```python
from build123d import *

# Parameters (mm, degrees)
ESBO_O1_R                = 18
RESSALTO_EXTRUS_O1_DEPTH = 3
RESSALTO_EXTRUS_O2_START = 5
RESSALTO_EXTRUS_O2_DEPTH = 5
RESSALTO_EXTRUS_O3_START = 2
RESSALTO_EXTRUS_O3_DEPTH = 2


with BuildPart() as part:
    # Esbo_o1 → Ressalto-extrus_o1 (new body)
    with BuildSketch(Plane.XY):
        with BuildLine():
            ThreePointArc((18, 0), (0, -18), (-18, 0))
            Line((-18, 0), (-18, 10.816653826))
            ThreePointArc((-18, 10.816653826), (-5.61248608, -20.236106345), (21, 0))
            ThreePointArc((21, 0), (20.236106345, 5.61248608), (18, 10.816653826))
            Line((18, 10.816653826), (18, 0))
        make_face()
        with BuildLine():
            Line((-18, 10.816653826), (-18, 0))
            ThreePointArc((-18, 0), (0, 18), (18, 0))
            Line((18, 0), (18, 10.816653826))
            ThreePointArc((18, 10.816653826), (0, 21), (-18, 10.816653826))
        make_face()
        Circle(ESBO_O1_R)
    extrude(amount=-RESSALTO_EXTRUS_O1_DEPTH)

    # Esbo_o1_3 → Ressalto-extrus_o2 (add)
    with BuildSketch(Plane.XY.offset(RESSALTO_EXTRUS_O2_START)):
        with BuildLine():
            ThreePointArc((18, 0), (0, -18), (-18, 0))
            Line((-18, 0), (-18, 10.816653826))
            ThreePointArc((-18, 10.816653826), (-5.61248608, -20.236106345), (21, 0))
            ThreePointArc((21, 0), (20.236106345, 5.61248608), (18, 10.816653826))
            Line((18, 10.816653826), (18, 0))
        make_face()
    extrude(amount=-RESSALTO_EXTRUS_O2_DEPTH)

    # Esbo_o3 → Ressalto-extrus_o3 (add)
    with BuildSketch(Plane.XY.offset(5).offset(RESSALTO_EXTRUS_O3_START)):
        with BuildLine():
            Line((-17, 0), (-17.419284402, 4.53525423))
            ThreePointArc((-17.419284402, 4.53525423), (-17.85423086, 2.286140937), (-18, 0))
            ThreePointArc((-18, 0), (0, -18), (18, 0))
            ThreePointArc((18, 0), (17.85423086, 2.286140937), (17.419284402, 4.53525423))
            Line((17.419284402, 4.53525423), (17, 0))
            ThreePointArc((17, 0), (0, -17), (-17, 0))
        make_face()
        with BuildLine():
            ThreePointArc((18, 0), (0, -18), (-18, 0))
            Line((-18, 0), (-18, 10.816653826))
            ThreePointArc((-18, 10.816653826), (0, -21), (18, 10.816653826))
            Line((18, 10.816653826), (18, 0))
        make_face()
        with BuildLine():
            Line((-17.419284402, 4.53525423), (-18, 10.816653826))
            Line((-18, 10.816653826), (-18, 0))
            ThreePointArc((-18, 0), (-17.85423086, 2.286140937), (-17.419284402, 4.53525423))
        make_face()
        with BuildLine():
            Line((18, 0), (18, 10.816653826))
            Line((18, 10.816653826), (17.419284402, 4.53525423))
            ThreePointArc((17.419284402, 4.53525423), (17.85423086, 2.286140937), (18, 0))
        make_face()
    extrude(amount=-RESSALTO_EXTRUS_O3_DEPTH)


solid = part.part
```
Input: part model. Units: mm. Frame: model coordinates. A direction names the side the tool comes from. Coordinates: 2 decimals unless noted, no trailing zeros. Loops run counter-clockwise (first coordinate to the right, second up) from the corner with the lowest first, then second, coordinate; pieces in that order, holes last. Notation, with made-up numbers: (-2, 20.5) -> (2, 20.5) arc R12 cw to (2, 29.5) -> close; hole circle Ø6 at (5.25, 45). An arc over 180 degrees is marked (long way). Use a Markdown table: item, result.
1) Pull-direction query (Z, two-part tool) for faces 1 (the cylindrical face through (0, -17, 6)), 2 (the flat face through (-1.4, -17.4, 5)), 3 (the flat face through (0, -18, 7)), 4 (the flat face through (0, 0, -3)); classes: released by +Z, released by -Z, zero draft, split by the parting line, or undercut.
Results found:
| item | result |
|---|---|
| face 1 | zero draft |
| face 2 | undercut |
| face 3 | released by +Z |
| face 4 | released by -Z |
2) Cut plane A-A (x = 0). Return the cut outline in (y, z), then the cut area to 3 significant figures.
Results found:
| item | result |
|---|---|
| outline | (-21, -3) -> (21, -3) -> (21, 0) -> (-18, 0) -> (-18, 5) -> (-17, 5) -> (-17, 7) -> (-21, 7) -> close |
| area | 149 mm2 |
3) Contact query for flat-ended pins moving along their axis: pin 1 (1.5 mm diameter, centred on x = -15.5, z = 1.5, fed in from -Y); pin 2 (1.5 mm diameter, centred on y = 7, z = 2.5, fed in from -X); pin 3 (11 mm diameter, centred on x = 7.5, y = -3.5, fed in from +Z). Output: stop coordinate, or through.
Results found:
| item | result |
|---|---|
| pin 1 | stops at y = -14.95 |
| pin 2 | stops at x = -20.05 |
| pin 3 | stops at z = 0 |
4) Access query for faces 5 (the cylindrical face through (0, -18, 3)), 6 (the cylindrical face through (3.522, -20.703, 2.07)). Directions: +Z, -Z, +X, -X, +Y, -Y. A direction counts if a zero-diameter tool reaches every point of the face in a straight line with its end or side. Return the directions, or none.
Results found:
| item | result |
|---|---|
| face 5 | +Y |
| face 6 | +Z, -Z |
5) Material intervals for line 1 along Z through (x, y) = (-4.5, -15); line 2 along X through (y, z) = (5, 0.75); line 3 along X through (y, z) = (-7.5, 4), sorted ascending. Write a range as from..to.
Results found:
| item | result |
|---|---|
| line 1 | z = -3..0 |
| line 2 | x = -20.4..-18, 18..20.4 |
| line 3 | x = -19.62..-16.36, 16.36..19.62 |
6) Cut plane B-B (z = 5.75). Return the cut outline in (x, y), then the cut area to 3 significant figures.
Results found:
| item | result |
|---|---|
| outline | (-18, 10.82) arc R21 ccw (long way) to (18, 10.82) -> (17, 0) arc R17 cw to (-17, 0) -> close |
| area | 294 mm2 |
7) Cut plane C-C (y = -0.5). Return the cut outline in (x, z).
Results found:
| item | result |
|---|---|
| outline | (-20.99, -3) -> (20.99, -3) -> (20.99, 7) -> (16.99, 7) -> (16.99, 5) -> (17.99, 5) -> (17.99, 0) -> (-17.99, 0) -> (-17.99, 5) -> (-16.99, 5) -> (-16.99, 7) -> (-20.99, 7) -> close |
8) Cut plane D-D (x = 10.5). Return the cut outline in (y, z).
Results found:
| item | result |
|---|---|
| outline | (-18.19, -3) -> (18.19, -3) -> (18.19, 0) -> (-14.62, 0) -> (-14.62, 5) -> (-13.37, 5) -> (-13.37, 7) -> (-18.19, 7) -> close |
